Design review of the part built by this model. Coordinates are the model's own, in mm. Coordinates: 2 decimals unless noted, no trailing zeros. Order: outer loops, then holes, each group sorted by start corner. A loop starts at its lowest first (then second) coordinate and runs counter-clockwise, first axis right, second up. Notation, with made-up numbers: M 12,49 L 16,49 A15 ccw 16,76 Z; hole C 45,-29.5 d4. An arc over 180 degrees is marked long. Answer as a JSON object with one key per item and string values.
from build123d import *

# Parameters (mm, degrees)
DOWN_BOARD_R    = 7.5
DOWN_BOARD_R_2  = 5
DOWN_BOARD_R_3  = 1.75
DOWN_BOARD_R_4  = 2.5
EXTRUDE_1_DEPTH = 1.5


with BuildPart() as part:
    # down_board → 凸台-拉伸1 (new body)
    with BuildSketch(Plane.XY):
        with BuildLine():
            Line((-65.577840697, 13.426839479), (-65.577840697, -13.426839479))
            ThreePointArc((-65.577840697, -13.426839479), (-64.116315672, -17.044296176), (-60.552102836, -18.631254027))
            Line((-60.552102836, -18.631254027), (-44.068912387, -18.631254027))
            Line((-44.068912387, -18.631254027), (-42.048007576, -20.229937109))
            Line((-42.048007576, -20.229937109), (-41.149136438, -21.908125258))
            Line((-41.149136438, -21.908125258), (-40.892469041, -23.789333182))
            Line((-40.892469041, -23.789333182), (-40.410773876, -26.102659685))
            Line((-40.410773876, -26.102659685), (-39.491433455, -28.071512622))
            Line((-39.491433455, -28.071512622), (-38.897523272, -28.966445774))
            Line((-38.897523272, -28.966445774), (-27.175557076, -40.560652421))
            Line((-27.175557076, -40.560652421), (-25.219810652, -40.800831807))
            Line((-25.219810652, -40.800831807), (-21.399814714, -40.800831807))
            Line((-21.399814714, -40.800831807), (-14.5, -38.99376786))
            Line((-14.5, -38.99376786), (-9.716490487, -38.215139203))
            Line((-9.716490487, -38.215139203), (-6.949583513, -38.111966401))
            Line((-6.949583513, -38.111966401), (-3.647583538, -38.009811446))
            Line((-3.647583538, -38.009811446), (1.739816686, -37.958836623))
            Line((1.739816686, -37.958836623), (7.734475924, -38.316671597))
            Line((7.734475924, -38.316671597), (17.40052023, -39.636214745))
            Line((17.40052023, -39.636214745), (21.017290997, -40.560652421))
            Line((21.017290997, -40.560652421), (23.930160234, -40.533091263))
            Line((23.930160234, -40.533091263), (25.930474181, -39.897299833))
            Line((25.930474181, -39.897299833), (27.847745393, -38.870371024))
            Line((27.847745393, -38.870371024), (29.373346844, -37.598162249))
            Line((29.373346844, -37.598162249), (31.356110551, -35.647675154))
            Line((31.356110551, -35.647675154), (38.246978904, -28.680874548))
            Line((38.246978904, -28.680874548), (39.890534987, -25.492625804))
            Line((39.890534987, -25.492625804), (40.133227927, -24.543113735))
            Line((40.133227927, -24.543113735), (40.347849385, -23.457827058))
            Line((40.347849385, -23.457827058), (40.559404219, -21.908125258))
            Line((40.559404219, -21.908125258), (40.559404219, -17.539392155))
            Line((40.559404219, -17.539392155), (41.168343616, -16.358142371))
            Line((41.168343616, -16.358142371), (42.790589116, -15.005341507))
            Line((42.790589116, -15.005341507), (45.499482621, -12.746377945))
            Line((45.499482621, -12.746377945), (46.605361545, -10.8932302))
            Line((46.605361545, -10.8932302), (46.605361545, 10.8932302))
            Line((46.605361545, 10.8932302), (45.499482621, 12.746377945))
            Line((45.499482621, 12.746377945), (42.790589116, 15.005341507))
            Line((42.790589116, 15.005341507), (41.168343616, 16.358142371))
            Line((41.168343616, 16.358142371), (40.559404219, 17.539392155))
            Line((40.559404219, 17.539392155), (40.559404219, 21.908125258))
            Line((40.559404219, 21.908125258), (40.347849385, 23.457827058))
            Line((40.347849385, 23.457827058), (40.133227927, 24.543113735))
            Line((40.133227927, 24.543113735), (39.890534987, 25.492625804))
            Line((39.890534987, 25.492625804), (38.246978904, 28.680874548))
            Line((38.246978904, 28.680874548), (31.356110551, 35.647675154))
            Line((31.356110551, 35.647675154), (29.373346844, 37.598162249))
            Line((29.373346844, 37.598162249), (27.847745393, 38.870371024))
            Line((27.847745393, 38.870371024), (25.930474181, 39.897299833))
            Line((25.930474181, 39.897299833), (23.930160234, 40.533091263))
            Line((23.930160234, 40.533091263), (21.017290997, 40.560652421))
            Line((21.017290997, 40.560652421), (17.40052023, 39.636214745))
            Line((17.40052023, 39.636214745), (7.734475924, 38.316671597))
            Line((7.734475924, 38.316671597), (1.739816686, 37.958836623))
            Line((1.739816686, 37.958836623), (-3.647583538, 38.009811446))
            Line((-3.647583538, 38.009811446), (-6.949583513, 38.111966401))
            Line((-6.949583513, 38.111966401), (-9.716490487, 38.215139203))
            Line((-9.716490487, 38.215139203), (-14.5, 38.99376786))
            Line((-14.5, 38.99376786), (-21.399814714, 40.800831807))
            Line((-21.399814714, 40.800831807), (-25.219810652, 40.800831807))
            Line((-25.219810652, 40.800831807), (-27.175557076, 40.560652421))
            Line((-27.175557076, 40.560652421), (-38.897523272, 28.966445774))
            Line((-38.897523272, 28.966445774), (-39.491433455, 28.071512622))
            Line((-39.491433455, 28.071512622), (-40.410773876, 26.102659685))
            Line((-40.410773876, 26.102659685), (-40.892469041, 23.789333182))
            Line((-40.892469041, 23.789333182), (-41.149136438, 21.908125258))
            Line((-41.149136438, 21.908125258), (-42.048007576, 20.229937109))
            Line((-42.048007576, 20.229937109), (-44.068912387, 18.631254027))
            Line((-44.068912387, 18.631254027), (-60.552102836, 18.631254027))
            ThreePointArc((-60.552102836, 18.631254027), (-64.116315672, 17.044296176), (-65.577840697, 13.426839479))
        make_face()
        with Locations((-29, 0)):
            Circle(DOWN_BOARD_R, mode=Mode.SUBTRACT)
        with Locations((29, 0)):
            Circle(DOWN_BOARD_R, mode=Mode.SUBTRACT)
        with Locations((-14.5, 29.5)):
            Circle(DOWN_BOARD_R_2, mode=Mode.SUBTRACT)
        with Locations(Location((14.5, 29.5, 0), (0, 0, 180))):
            Circle(DOWN_BOARD_R_2, mode=Mode.SUBTRACT)
        with Locations((14.5, -29.5)):
            Circle(DOWN_BOARD_R_2, mode=Mode.SUBTRACT)
        with Locations(Location((-14.5, -29.5, 0), (0, 0, 180))):
            Circle(DOWN_BOARD_R_2, mode=Mode.SUBTRACT)
        with Locations((-36.75, 26.25)):
            Circle(DOWN_BOARD_R_3, mode=Mode.SUBTRACT)
        with Locations((-26.143398282, 36.856601718)):
            Circle(DOWN_BOARD_R_3, mode=Mode.SUBTRACT)
        with Locations(Location((36.75, 26.25, 0), (0, 0, 180))):
            Circle(DOWN_BOARD_R_3, mode=Mode.SUBTRACT)
        with Locations(Location((26.143398282, 36.856601718, 0), (0, 0, 180))):
            Circle(DOWN_BOARD_R_3, mode=Mode.SUBTRACT)
        with Locations((36.75, -26.25)):
            Circle(DOWN_BOARD_R_3, mode=Mode.SUBTRACT)
        with Locations((26.143398282, -36.856601718)):
            Circle(DOWN_BOARD_R_3, mode=Mode.SUBTRACT)
        with Locations(Location((-36.75, -26.25, 0), (0, 0, 180))):
            Circle(DOWN_BOARD_R_3, mode=Mode.SUBTRACT)
        with Locations(Location((-26.143398282, -36.856601718, 0), (0, 0, 180))):
            Circle(DOWN_BOARD_R_3, mode=Mode.SUBTRACT)
        with Locations((0, -30.5)):
            Circle(DOWN_BOARD_R_4, mode=Mode.SUBTRACT)
        with Locations(Location((0, 30.5, 0), (0, 0, 180))):
            Circle(DOWN_BOARD_R_4, mode=Mode.SUBTRACT)
        with BuildLine():
            Line((-9, -15), (9, -15))
            ThreePointArc((9, -15), (11, -17), (9, -19))
            Line((9, -19), (-9, -19))
            ThreePointArc((-9, -19), (-11, -17), (-9, -15))
        make_face(mode=Mode.SUBTRACT)
        with BuildLine():
            Line((-12.5, 2), (12.5, 2))
            ThreePointArc((12.5, 2), (14.5, 0), (12.5, -2))
            Line((12.5, -2), (-12.5, -2))
            ThreePointArc((-12.5, -2), (-14.5, 0), (-12.5, 2))
        make_face(mode=Mode.SUBTRACT)
        with BuildLine():
            Line((-9, 15), (9, 15))
            ThreePointArc((9, 15), (11, 17), (9, 19))
            Line((9, 19), (-9, 19))
            ThreePointArc((-9, 19), (-11, 17), (-9, 15))
        make_face(mode=Mode.SUBTRACT)
        with BuildLine():
            Line((41.5, -4.5), (41.5, 4.5))
            ThreePointArc((41.5, 4.5), (42.5, 5.5), (43.5, 4.5))
            Line((43.5, 4.5), (43.5, -4.5))
            ThreePointArc((43.5, -4.5), (42.5, -5.5), (41.5, -4.5))
        make_face(mode=Mode.SUBTRACT)
    extrude(amount=EXTRUDE_1_DEPTH)


solid = part.part
1) Add section C-C (x = -59). State the section outline as (y, z) points, and give its area (3 significant figures).
Taken from the geometry:
{"outline": "M -18.63,0 L 18.63,0 L 18.63,1.5 L -18.63,1.5 Z", "area": "55.9 mm2"}
2) Mouldability with a two-part tool opening along Y and no side actions: class faces 1 (the cylindrical face through (26.523, 38.565, 0.74)), 2 (the flat face through (-10, -8, 0)), 3 (the flat face through (-33, 34.8, 0.7)) as released by +Y, released by -Y, zero draft, split by the parting line, or undercut.
Taken from the geometry:
{"face 1": "undercut", "face 2": "zero draft", "face 3": "released by +Y"}
3) To check wall thickness, follow L1, parallel to Y at x = -6.5, z = 0.85; L2, parallel to Y at x = 1.5, z = 1.3; L3, parallel to Y at x = 12, z = 1.3. State the ranges of each line that lie inside material, in increasing order.
Taken from the geometry:
{"L1": "y = -38.1 to -19, -15 to -2, 2 to 15, 19 to 38.1", "L2": "y = -37.96 to -32.5, -28.5 to -19, -15 to -2, 2 to 15, 19 to 28.5, 32.5 to 37.96", "L3": "y = -38.9 to -33.83, -25.17 to -2, 2 to 25.17, 33.83 to 38.9"}
4) Add section D-D (z = 0.3). Count the separate pieces of the cut face and the enclosed holes in it, and give its area (3 significant figures).
Taken from the geometry:
{"separate pieces": "1", "enclosed holes": "20", "area": "6,060 mm2"}
5) Insertion check: pin 1 Ø2 at (x, y) = (-26.14, -36.86) entering from +Z; pin 2 Ø0.8 at (x, z) = (2.5, 1) entering from -Y. Each pin has a flat end and moves straight along its axis. Give the tip position at first contact, or say it passes through.
Taken from the geometry:
{"pin 1": "passes through", "pin 2": "stops at y = -38.03"}
6) Add section A-A (x = -23). State the section outline as (y, z) points, and give its area (3 significant figures).
Taken from the geometry:
{"outline": "M -40.8,0 L -4.5,0 L -4.5,1.5 L -40.8,1.5 Z; M 4.5,0 L 40.8,0 L 40.8,1.5 L 4.5,1.5 Z", "area": "109 mm2"}
7) Add section B-B (y = 0). State the section outline as (x, z) points.
Taken from the geometry:
{"outline": "M -65.58,0 L -36.5,0 L -36.5,1.5 L -65.58,1.5 Z; M -21.5,0 L -14.5,0 L -14.5,1.5 L -21.5,1.5 Z; M 14.5,0 L 21.5,0 L 21.5,1.5 L 14.5,1.5 Z; M 36.5,0 L 41.5,0 L 41.5,1.5 L 36.5,1.5 Z; M 43.5,0 L 46.61,0 L 46.61,1.5 L 43.5,1.5 Z"}
